from build123d import *

# Parameters (mm, degrees)
SKETCH2_R = 0.762


with BuildPart() as part:
    # Base-Sweep: sweep along a path in Sketch1
    with BuildLine(Plane.XY) as base_sweep_path:
        Line((-1.143, 0), (1.143, 0))
        ThreePointArc((1.143, 0), (2.759446102, 0.669553898), (3.429, 2.286))
        Line((3.429, 2.286), (3.429, 10.16))
        Line((3.429, 10.16), (2.461534374, 13.961457123))
        ThreePointArc((2.461534374, 13.961457123), (0, 15.875), (-2.461534374, 13.961457123))
        Line((-2.461534374, 13.961457123), (-3.429, 10.16))
        Line((-3.429, 10.16), (-3.429, 2.286))
        ThreePointArc((-3.429, 2.286), (-2.759446102, 0.669553898), (-1.143, 0))
    # Sketch2 → Base-Sweep (sweep)
    with BuildSketch(Plane(origin=(0, 0, 0), x_dir=(0, 0, -1), z_dir=(1, 0, 0))):
        Circle(SKETCH2_R)
    sweep(path=base_sweep_path.line, transition=Transition.RIGHT)


solid = part.part
Work out the finished part from the listing and answer in its coordinate system (mm). Coordinates: 2 decimals unless noted, no trailing zeros. Write each loop counter-clockwise with the first axis right and the second up, starting at its lowest first coordinate (ties: lowest second). Pieces come first, ordered by that corner, then holes.
1. Consider line 1 along Y through (x, z) = (1, -0.6); line 2 along Y through (x, z) = (1.5, 0.45); line 3 along X through (y, z) = (13, 0.25). Determine where each line is inside the solid, lowest interval first.
Results list:
line 1: y = -0.47 to 0.47, 15.15 to 16.17
line 2: y = -0.59 to 0.65, 14.54 to 16.11
line 3: x = -3.45 to -1.96, 1.96 to 3.45
2. The part is cut by section B-B, the plane y = 6. Write down the section's boundary in (x, z).
Results list:
outline: circle Ø1.52 at (-3.43, 0); circle Ø1.52 at (3.43, 0)
3. The part is cut by section A-A, the plane z = 0. Write down the section's boundary in (x, y) (3 decimals), and give its area (3 significant figures).
Results list:
outline: (-4.191, 2.286) arc R3.048 ccw to (-1.143, -0.762) - (1.143, -0.762) arc R3.048 ccw to (4.191, 2.286) - (4.191, 10.255) - (3.2, 14.149) arc R3.302 ccw to (-3.2, 14.149) - (-4.191, 10.255) - close; hole (-2.667, 2.286) arc R1.524 ccw to (-1.143, 0.762) - (1.143, 0.762) arc R1.524 ccw to (2.667, 2.286) - (2.667, 10.065) - (1.723, 13.774) arc R1.778 ccw to (-1.723, 13.774) - (-2.667, 10.065) - close
area: 60.6 mm2
